```python
from build123d import *

# Parameters (mm, degrees)
EXTRUDE_1_DEPTH     = 3
SKETCH_2_W          = 17.5
SKETCH_2_H          = 13
CUT_EXTRUDE_1_DEPTH = 41.443247314
EXTRUDE_2_DEPTH     = 20


with BuildPart() as part:
    # Эскиз1 → Бобышка-Вытянуть1 (new body)
    with BuildSketch(Plane(origin=(0, 0, 0), x_dir=(1, 0, 0), z_dir=(0, 1, 0))):
        Polygon((0, 0), (30, 0), (35.02365277, -20), (5.02365277, -20), align=None)
    extrude(amount=EXTRUDE_1_DEPTH)

    # Эскиз2 → Вырез-Вытянуть1 (cut, through all)
    with BuildSketch(Plane(origin=(0, 3, 0), x_dir=(1, 0, 0), z_dir=(0, 1, 0))):
        with Locations((17.511826385, -10)):
            Rectangle(SKETCH_2_W, SKETCH_2_H)
    extrude(amount=-CUT_EXTRUDE_1_DEPTH, mode=Mode.SUBTRACT)

    # Эскиз3 → Бобышка-Вытянуть2 (add)
    with BuildSketch(Plane.XZ):
        Polygon((5.02365277, 20), (0, 0), (30, 0), (35.02365277, 20), align=None)
        Polygon((6.583415246, 18), (2.56449303, 2), (28.440237524, 2), (32.459159739, 18), align=None, mode=Mode.SUBTRACT)
    extrude(amount=EXTRUDE_2_DEPTH)


solid = part.part
```
The model under review builds one solid part; all positions refer to its coordinate system, in mm. A direction names the side the tool comes from. Coordinates: 2 decimals unless noted, no trailing zeros. Write each loop counter-clockwise with the first axis right and the second up, starting at its lowest first coordinate (ties: lowest second). Pieces come first, ordered by that corner, then holes. Notation, with made-up numbers: (79, 8) - (115, 8) arc R23 ccw to (115, 20) - close; hole circle Ø9 at (-28, -13). An arc over 180 degrees is marked (long way). Write item = value, one per line.
(1) Consider section D-D, the plane x = 7.5. Give the boundary of the cut face in (y, z), then the cut area to 3 significant figures.
Result sheet:
outline = (-20, 0) - (3, 0) - (3, 20) - (-20, 20) - (-20, 18) - (0, 18) - (0, 2) - (-20, 2) - close
area = 140 mm^2
(2) For line 1 (Z direction, x = 22, y = -3.25); line 2 (Z direction, x = 13, y = 0.75); line 3 (X direction, y = 1.75, z = 7.5), list the stretches that pass through material, from the lowest coordinate up. Write a range as [from, to].
Result sheet:
line_1 = [0, 2], [18, 20]
line_2 = [0, 3.5], [16.5, 20]
line_3 = [1.88, 8.76], [26.26, 31.88]
(3) Consider section B-B, the plane z = 9.75. Give the boundary of the cut face in (x, y).
Result sheet:
outline = (2.45, -20) - (4.51, -20) - (4.51, 0) - (8.76, 0) - (8.76, 3) - (2.45, 3) - close; (26.26, 0) - (30.39, 0) - (30.39, -20) - (32.45, -20) - (32.45, 3) - (26.26, 3) - close
(4) Consider section A-A, the plane x = 23.5. Give the boundary of the cut face in (y, z), then the cut area to 3 significant figures.
Result sheet:
outline = (-20, 0) - (3, 0) - (3, 3.5) - (0, 3.5) - (0, 2) - (-20, 2) - close; (-20, 18) - (0, 18) - (0, 16.5) - (3, 16.5) - (3, 20) - (-20, 20) - close
area = 101 mm^2
(5) Machinability: for faces 4 (the face through (26.262, 2, 10)), 5 (the face through (4.6, -9.9, 10.1)), 6 (the face through (32.477, -8.339, 9.86)), which of the approach directions +Z, -Z, +X, -X, +Y, -Y give a long, thin tool a straight path to every point of the face, cutting with its end or side? Answer none if there is none.
Result sheet:
face_4 = +Y, -Y
face_5 = -Y
face_6 = -Z, +X, +Y, -Y
(6) For P1, Ø2, axis at y = -9, z = 4.5, coming from the +X side; P2, Ø3.5, axis at x = 13.5, y = 1, coming from the -Z side; P3, Ø1, axis at y = -10, z = 13.5, coming from the +X side; P4, Ø3, axis at x = 10.5, z = 11.5, coming from the -Y side, all flat-tipped, find the tip position at first contact; note any pin that passes through.
Result sheet:
P1 = 31.38
P2 = 0
P3 = 33.52
P4 = through
(7) Consider section C-C, the plane y = -5.25. Give the boundary of the cut face in (x, z).
Result sheet:
outline = (0, 0) - (30, 0) - (35.02, 20) - (5.02, 20) - close; hole (2.56, 2) - (28.44, 2) - (32.46, 18) - (6.58, 18) - close
(8) Mouldability with a two-part tool opening along Z and no side actions: class faces 1 (the face through (18, 0, 3)), 2 (the face through (18, 3, 3)), 3 (the face through (15, -8, 0)) as pulls with the +Z half, pulls with the -Z half, needs draft (parallel to the pull), parting line crosses it, or undercut.
Result sheet:
face_1 = undercut
face_2 = needs draft
face_3 = pulls with the -Z half
